Could you check a few things on this model? Use its own coordinates, in mm. Round coordinates to 2 decimals unless told otherwise and drop trailing zeros. Loops run counter-clockwise (first coordinate to the right, second up) from the corner with the lowest first, then second, coordinate; pieces in that order, holes last. Notation, with made-up numbers: (51.5, -15) - (110.5, -15) arc R18 ccw to (110.5, -5) - close; hole circle Ø5 at (-20.5, 54). An arc over 180 degrees is marked (long way). Use one line per item in the form item = value.
Autodesk Inventor part; units mm, degrees
ref_plane "YZ Plane" through (0, 0, 0) normal (1, 0, 0) x (0, 1, 0)
ref_plane "XZ Plane" through (0, 0, 0) normal (0, 1, 0) x (-1, 0, 0)
ref_plane "XY Plane" through (0, 0, 0) normal (0, 0, 1) x (1, 0, 0)
sketch "Sketch1" plane through (0, 0, 0) normal (0, 0, 1) x (1, 0, 0)
  line L0 (-12.7, -12.7) -> (-12.7, 12.7)
  line L1 (-12.7, 12.7) -> (12.7, 12.7)
  line L2 (12.7, 12.7) -> (12.7, -12.7)
  line L3 (12.7, -12.7) -> (-12.7, -12.7)
  line L4 (-12.7, -12.7) -> (12.7, 12.7) construction
  line L5 (-12.7, 12.7) -> (12.7, -12.7) construction
  line L6 (11.1125, 11.1125) -> (-11.1125, 11.1125)
  line L7 (-11.1125, 11.1125) -> (-11.1125, -11.1125)
  line L8 (-11.1125, -11.1125) -> (11.1125, -11.1125)
  line L9 (11.1125, -11.1125) -> (11.1125, 11.1125)
  point P0 (0, 0)
  dimension "d0" = 25.4
  dimension "d1" = 25.4
  dimension "d2" = 1.5875
extrude "Extrusion1" add sketch "Sketch1" along normal blind 355.6
equation "\"d1\" = d0"
properties part number "14in long 1in square tube"
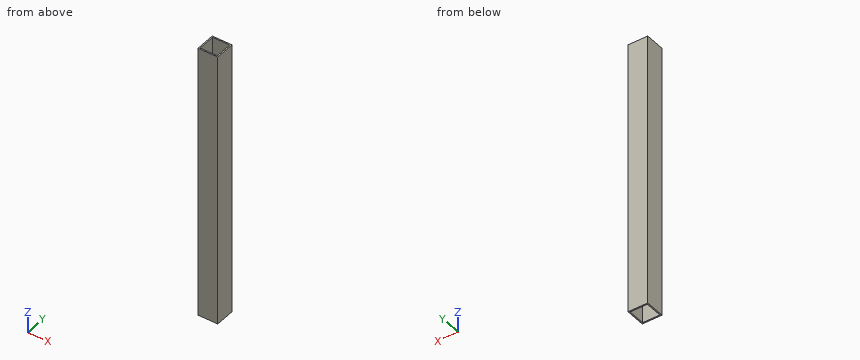
1. If we section it at C-C, the plane z = 188.5: Write out the boundary of the cut face in (x, y).
Solution:
outline = (-12.7, -12.7) - (12.7, -12.7) - (12.7, 12.7) - (-12.7, 12.7) - close; hole (-11.11, -11.11) - (11.11, -11.11) - (11.11, 11.11) - (-11.11, 11.11) - close
2. Please list where this line runs through material, in increasing order: line 1 along X through (y, z) = (5.75, 202).
Solution:
line_1 = -12.7 to -11.11, 11.11 to 12.7
3. If we section it at A-A, the plane y = -2.75: Write out the boundary of the cut face in (x, z), plus the area to 3 significant figures.
Solution:
outline = (-12.7, 0) - (-11.11, 0) - (-11.11, 355.6) - (-12.7, 355.6) - close; (11.11, 0) - (12.7, 0) - (12.7, 355.6) - (11.11, 355.6) - close
area = 1,130 mm^2
